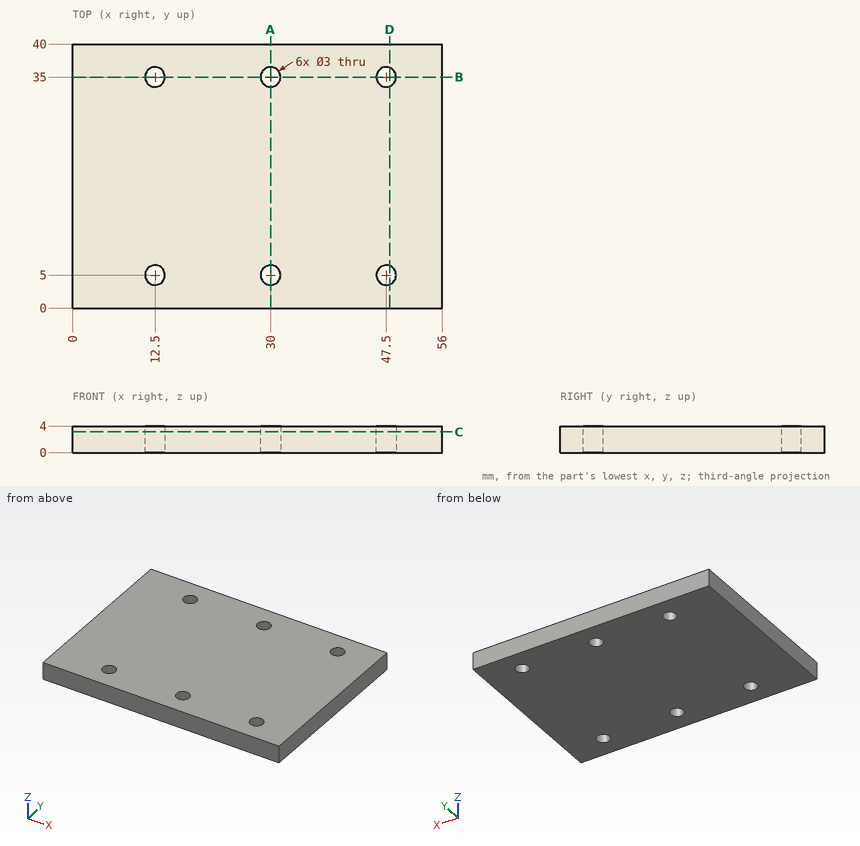
Geometry check sheet. Reference: drawing and pictorial views, mm from the part's lowest x, y, z. Round coordinates to 2 decimals unless told otherwise and drop trailing zeros. Write each loop counter-clockwise with the first axis right and the second up, starting at its lowest first coordinate (ties: lowest second). Pieces come first, ordered by that corner, then holes.
1. Scan lines: L1, parallel to Y at x = 12.5, z = 3.1; L2, parallel to Y at x = 46.5, z = 2.45. Record each from-to range of solid material in increasing order.
2. Section check D-D on x = 48. Enter the section's corners in (y, z), plus the area to 3 significant figures.
3. Gauge pin test, flat end, axial feed: P1, Ø2.5, axis at x = 30, y = 35, coming from the +Z side. Record the tip position at first contact, or that the pin passes through.
4. Section check B-B on y = 35. Enter the section's corners in (x, z), plus the area to 3 significant figures.
5. Section check C-C on z = 3.15. Enter the section's corners in (x, y).
6. Section check A-A on x = 30. Enter the section's corners in (y, z), plus the area to 3 significant figures.
Answer:
1. L1: y = 0 to 3.5, 6.5 to 33.5, 36.5 to 40
1. L2: y = 0 to 3.88, 6.12 to 33.88, 36.12 to 40
2. outline: (0, 0) - (3.59, 0) - (3.59, 4) - (0, 4) - close; (6.41, 0) - (33.59, 0) - (33.59, 4) - (6.41, 4) - close; (36.41, 0) - (40, 0) - (40, 4) - (36.41, 4) - close
2. area: 137 mm2
3. P1: passes through
4. outline: (0, 0) - (11, 0) - (11, 4) - (0, 4) - close; (14, 0) - (28.5, 0) - (28.5, 4) - (14, 4) - close; (31.5, 0) - (46, 0) - (46, 4) - (31.5, 4) - close; (49, 0) - (56, 0) - (56, 4) - (49, 4) - close
4. area: 188 mm2
5. outline: (0, 0) - (56, 0) - (56, 40) - (0, 40) - close; hole circle Ø3 at (12.5, 5); hole circle Ø3 at (12.5, 35); hole circle Ø3 at (30, 5); hole circle Ø3 at (30, 35); hole circle Ø3 at (47.5, 5); hole circle Ø3 at (47.5, 35)
6. outline: (0, 0) - (3.5, 0) - (3.5, 4) - (0, 4) - close; (6.5, 0) - (33.5, 0) - (33.5, 4) - (6.5, 4) - close; (36.5, 0) - (40, 0) - (40, 4) - (36.5, 4) - close
6. area: 136 mm2
